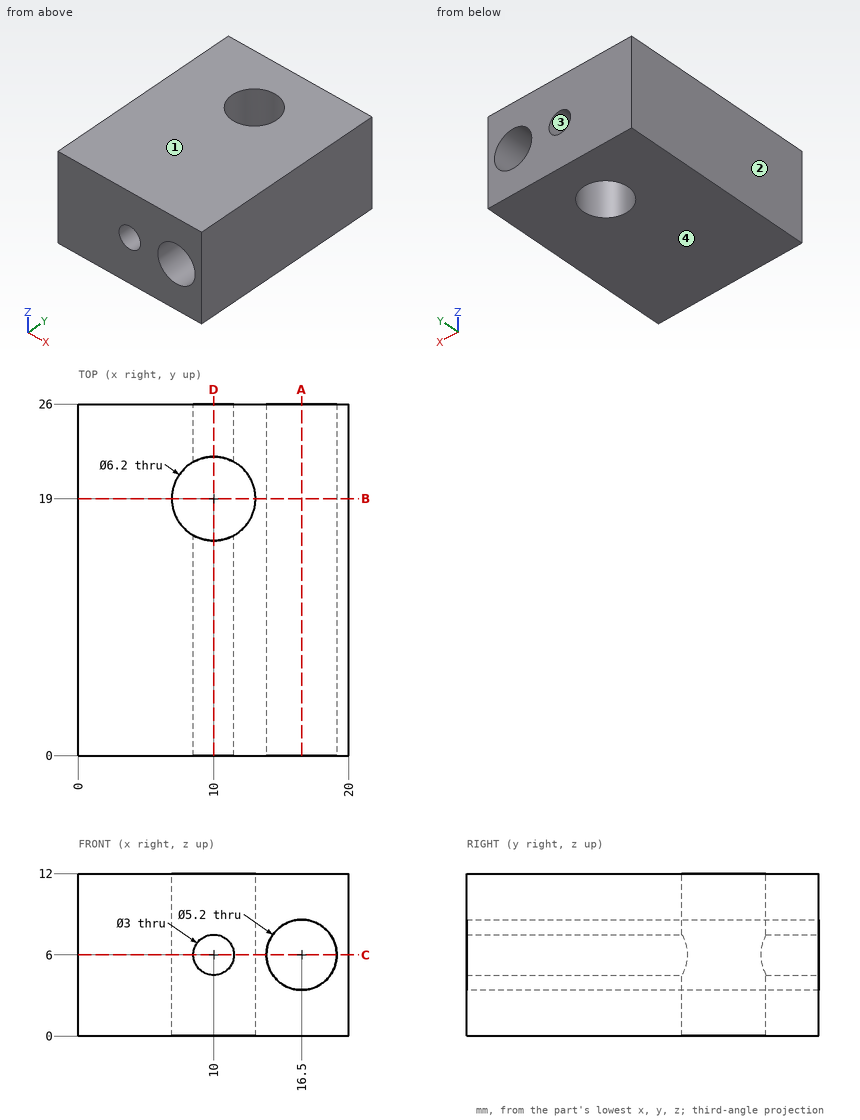
Design review of the part shown in the three views and the two pictorial views. Dimensions are in mm from the part's minimum x, y and z. Give positions to 0.01 mm unless a question says otherwise; leave off trailing zeros. Write each loop counter-clockwise with the first axis right and the second up, starting at its lowest first coordinate (ties: lowest second). Pieces come first, ordered by that corner, then holes. Notation, with made-up numbers: (73, 54.25) -> (92, 54.25) arc R28 ccw to (92, 82.25) -> close; hole circle Ø1 at (45, -18.5). An arc over 180 degrees is marked (long way). Answer in a Markdown table with one row per item.
1) Add section B-B on y = 19. State the section outline as (x, z) points.
Worked answers:
| item | result |
|---|---|
| outline | (0, 0) -> (6.9, 0) -> (6.9, 12) -> (0, 12) -> close; (13.1, 0) -> (20, 0) -> (20, 12) -> (13.1, 12) -> close; hole circle Ø5.2 at (16.5, 6) |
2) Add section A-A on x = 16.5. State the section outline as (y, z) points.
Worked answers:
| item | result |
|---|---|
| outline | (0, 0) -> (26, 0) -> (26, 3.4) -> (0, 3.4) -> close; (0, 8.6) -> (26, 8.6) -> (26, 12) -> (0, 12) -> close |
3) Add section C-C on z = 6. State the section outline as (x, y) points, plus the area to 3 significant figures.
Worked answers:
| item | result |
|---|---|
| outline | (0, 0) -> (8.5, 0) -> (8.5, 16.29) arc R3.1 cw to (8.5, 21.71) -> (8.5, 26) -> (0, 26) -> close; (11.5, 0) -> (13.9, 0) -> (13.9, 26) -> (11.5, 26) -> (11.5, 21.71) arc R3.1 cw to (11.5, 16.29) -> close; (19.1, 0) -> (20, 0) -> (20, 26) -> (19.1, 26) -> close |
| area | 294 mm² |
4) For L1, parallel to X at y = 16.25, z = 6; L2, parallel to Z at x = 10, y = 12; L3, parallel to Y at x = 10, z = 8, list the stretches that pass through material, from the lowest coordinate up. Write a range as [from, to].
Worked answers:
| item | result |
|---|---|
| L1 | [0, 8.5], [11.5, 13.9], [19.1, 20] |
| L2 | [0, 4.5], [7.5, 12] |
| L3 | [0, 15.9], [22.1, 26] |
5) Add section D-D on x = 10. State the section outline as (y, z) points.
Worked answers:
| item | result |
|---|---|
| outline | (0, 0) -> (15.9, 0) -> (15.9, 4.5) -> (0, 4.5) -> close; (0, 7.5) -> (15.9, 7.5) -> (15.9, 12) -> (0, 12) -> close; (22.1, 0) -> (26, 0) -> (26, 4.5) -> (22.1, 4.5) -> close; (22.1, 7.5) -> (26, 7.5) -> (26, 12) -> (22.1, 12) -> close |
6) Mouldability with a two-part tool opening along Z and no side actions: class the marked faces 1, 2, 3 and 4 as +Z half, -Z half, draft (parallel to the pull), parting line (faces both ways), or undercut.
Worked answers:
| item | result |
|---|---|
| face 1 | +Z half |
| face 2 | draft |
| face 3 | undercut |
| face 4 | -Z half |
